Input: dimensioned drawing with shaded views. Units: mm. Origin: part minimum x, y, z. A direction names the side the tool comes from. Give positions to 0.01 mm unless a question says otherwise; leave off trailing zeros. Order: outer loops, then holes, each group sorted by start corner. A loop starts at its lowest first (then second) coordinate and runs counter-clockwise, first axis right, second up.
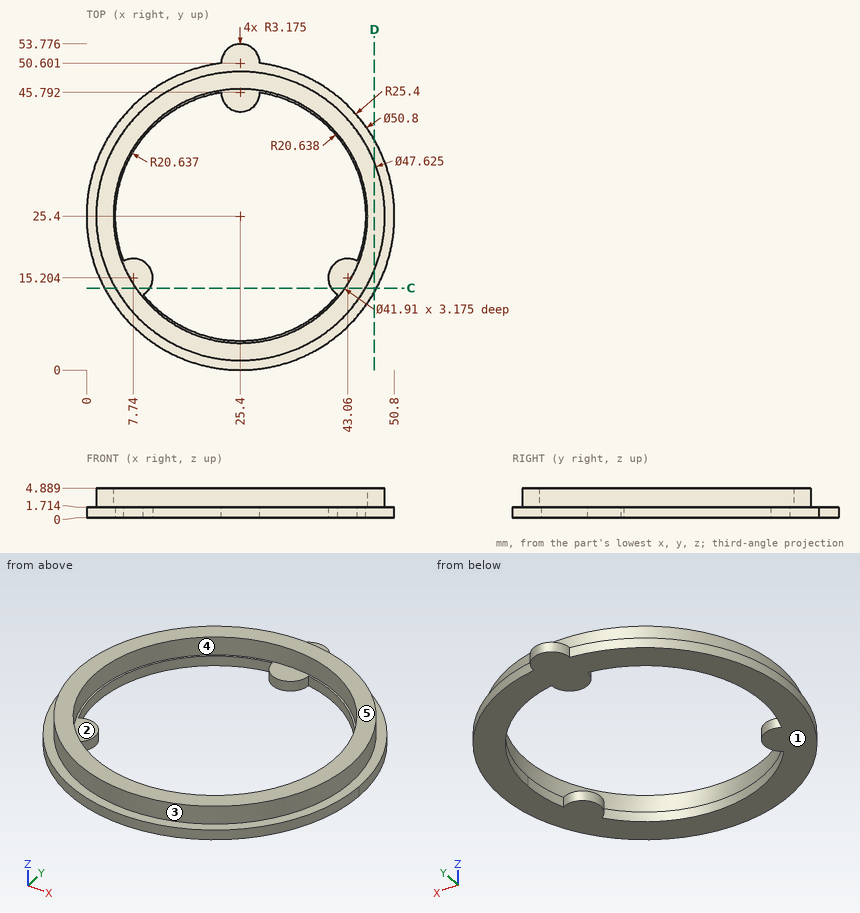
1) Pin query (flat end, axial travel): pin 1 (2 mm diameter, centred on x = 7.5, z = 3.5, fed in from -Y) (1 decimal); pin 2 (1 mm diameter, centred on y = 34.5, z = 3, fed in from +X) (1 decimal); pin 3 (2 mm diameter, centred on x = 42, z = 3, fed in from +Y). Return the tip coordinate at first contact, or that it passes through.
Report:
pin 1: stops at y = 8.6
pin 2: stops at x = 47.6
pin 3: stops at y = 43.39
2) Section query C-C, the plane y = 13.5. Return the cut outline in (x, z) (1 decimal).
Report:
outline: (3, 0) - (10.4, 0) - (10.4, 1.7) - (8.2, 1.7) - (8.2, 4.9) - (4.8, 4.9) - (4.8, 1.7) - (3, 1.7) - close; (40.4, 0) - (47.8, 0) - (47.8, 1.7) - (46, 1.7) - (46, 4.9) - (42.6, 4.9) - (42.6, 1.7) - (40.4, 1.7) - close
3) Reachability of the marked faces 1 and 2 from +Z, -Z, +X, -X, +Y, -Y: full face, straight path, thin tool, end or side. Return the list, or none.
Report:
face 1: -Z, +X, -X, +Y, -Y
face 2: +Z
4) Draft query along Y for the marked faces 3, 4 and 5. Return one class per face: +Y half, -Y half, draft (parallel to the pull), parting line (faces both ways), or undercut.
Report:
face 3: parting line
face 4: undercut
face 5: draft
5) Section query D-D, the plane x = 47.5. Return the cut outline in (y, z) (1 decimal).
Report:
outline: (12.9, 0) - (37.9, 0) - (37.9, 1.7) - (34.3, 1.7) - (34.3, 4.9) - (16.5, 4.9) - (16.5, 1.7) - (12.9, 1.7) - close
6) Material intervals for L1, parallel to Y at x = 25.4, z = 3.05 (1 decimal); L2, parallel to X at y = 39.5, z = 4.3; L3, parallel to Y at x = 7.5, z = 3.6 (1 decimal), sorted ascending.
Report:
L1: y = 1.6 to 4.4, 46.4 to 49.2
L2: x = 6.21 to 9.9, 40.9 to 44.59
L3: y = 9.7 to 14.5, 36.3 to 41.1
